Answer from the drawing. Dimensions are ordinates in mm from the lowest x, y and z of the part. Coordinates: 2 decimals unless noted, no trailing zeros. Write each loop counter-clockwise with the first axis right and the second up, starting at its lowest first coordinate (ties: lowest second). Pieces come first, ordered by that corner, then holes.
(1) The part is cut by section B-B on x = 146.05. Determine the outline of the cut face in (y, z) (3 decimals).
(2) Straight lines are drawn through the part: line 1 (X direction, y = 6, z = 5.25); line 2 (Y direction, x = 146.05, z = 3) (3 decimals); line 3 (Y direction, x = 39, z = 5.25). For each, find the intervals that lie inside material, in ascending order.
(3) Given P1, Ø3.5, axis at x = 38.1, y = 50.8, coming from the +Z side, flat-ended and moving along its own axis, determine where the tip first touches the part or whether it passes through.
(4) The part is cut by section C-C on x = 38.1. Determine the outline of the cut face in (y, z) (3 decimals).
(5) The part is cut by section A-A on y = 6.35. Determine the outline of the cut face in (x, z) (3 decimals), plus the area to 3 significant figures.
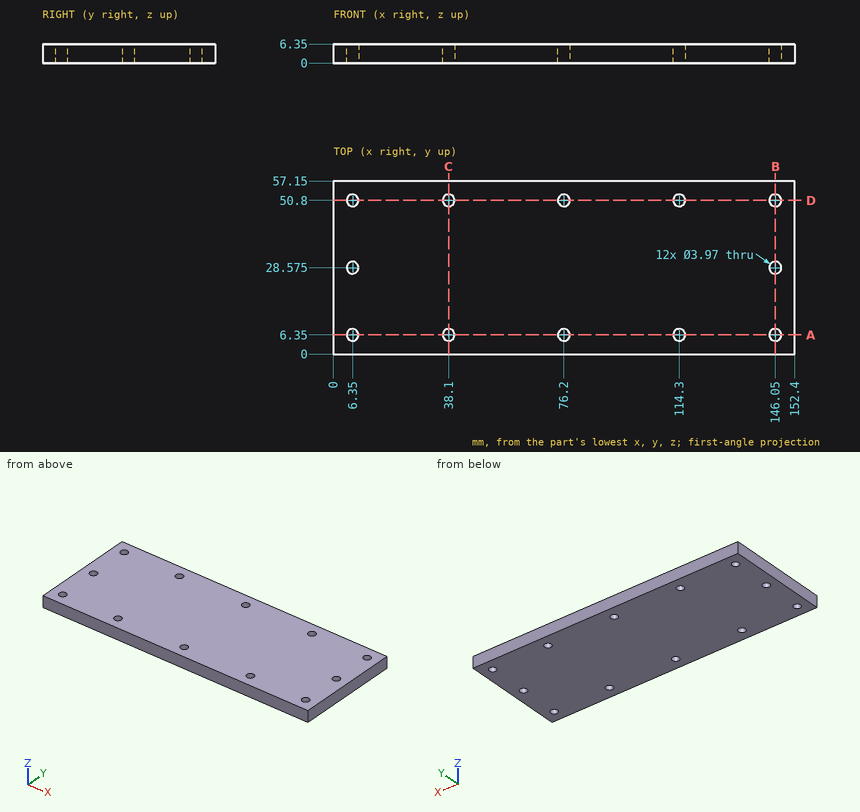
Model answer:
1. outline: (0, 0) - (4.365, 0) - (4.365, 6.35) - (0, 6.35) - close; (8.335, 0) - (26.59, 0) - (26.59, 6.35) - (8.335, 6.35) - close; (30.56, 0) - (48.815, 0) - (48.815, 6.35) - (30.56, 6.35) - close; (52.785, 0) - (57.15, 0) - (57.15, 6.35) - (52.785, 6.35) - close
2. line 1: x = 0 to 4.4, 8.3 to 36.15, 40.05 to 74.25, 78.15 to 112.35, 116.25 to 144.1, 148 to 152.4
2. line 2: y = 0 to 4.365, 8.335 to 26.59, 30.56 to 48.815, 52.785 to 57.15
2. line 3: y = 0 to 4.58, 8.12 to 49.03, 52.57 to 57.15
3. P1: passes through
4. outline: (0, 0) - (4.365, 0) - (4.365, 6.35) - (0, 6.35) - close; (8.335, 0) - (48.815, 0) - (48.815, 6.35) - (8.335, 6.35) - close; (52.785, 0) - (57.15, 0) - (57.15, 6.35) - (52.785, 6.35) - close
5. outline: (0, 0) - (4.365, 0) - (4.365, 6.35) - (0, 6.35) - close; (8.335, 0) - (36.115, 0) - (36.115, 6.35) - (8.335, 6.35) - close; (40.085, 0) - (74.215, 0) - (74.215, 6.35) - (40.085, 6.35) - close; (78.185, 0) - (112.315, 0) - (112.315, 6.35) - (78.185, 6.35) - close; (116.285, 0) - (144.065, 0) - (144.065, 6.35) - (116.285, 6.35) - close; (148.035, 0) - (152.4, 0) - (152.4, 6.35) - (148.035, 6.35) - close
5. area: 842 mm2
